from build123d import *


with BuildPart() as f1:
    # F0 (on Front) → F1 (revolve)
    with BuildSketch(Plane.XZ):
        Polygon((17.880435, -35.012588), (0, -35.012588), (0, -38.822588), (20.221465, -38.822588), align=None)
        with BuildLine():
            ThreePointArc((26.210172, 7.225862), (25.094249, 9.919939), (22.400172, 11.035862))
            Line((22.400172, 11.035862), (18.590172, 7.225862))
            Line((18.590172, 7.225862), (18.590172, -12.52082))
            Line((18.590172, -12.52082), (26.210172, -8.298599))
            Line((26.210172, -8.298599), (26.210172, 7.225862))
        make_face()
        Polygon((18.590172, -12.52082), (18.590172, 7.225862), (3.823765, -9.549403), (3.823765, -23.782769), (0, -28.126729), (0, -35.012588), (17.880435, -35.012588), (13.834589, -28.428022), (13.834589, -15.155875), align=None)
    revolve(axis=Axis((0, 0, -13.893363), (0, 0, -1)))


solid = f1.part
Verification items for the finished model (mm, model axes). A direction names the side the tool comes from. Coordinates: 2 decimals unless noted, no trailing zeros. Loops run counter-clockwise (first coordinate to the right, second up) from the corner with the lowest first, then second, coordinate; pieces in that order, holes last. Notation, with made-up numbers: (53.25, 53.5) -> (79.25, 53.5) arc R27 ccw to (79.25, 72.5) -> close; hole circle Ø8 at (16.5, -40). An arc over 180 degrees is marked (long way). Answer as a JSON object with one key per item and string values. Group by question number.
Item 1: Tool access check on faces 1 (the cylindrical face through (13.196, -4.156, -21.699)), 2 (the cylindrical face through (-0.829, 3.733, -16.766)). Record the directions out of +Z, -Z, +X, -X, +Y, -Y that give a thin tool (end or side, any length) a straight path to the whole face; none if there is none.
Item 2: Depth check by flat-ended pin: pin 1 (1.5 mm diameter, centred on y = -15, z = -3.5, fed in from -X); pin 2 (3 mm diameter, centred on y = -3, z = -22.5, fed in from -X); pin 3 (6 mm diameter, centred on y = -14, z = -30.5, fed in from +X). Enter the tip coordinate at first touch or a pass-through.
Item 3: Sectioned sample at B-B on z = -31. Record the boundary of the cut face in (x, y).
Item 4: Sectioned sample at A-A on z = -26. Record the boundary of the cut face in (x, y), plus the area to 3 significant figures.
Item 5: Mould release check, pull along X, two halves, no side actions. Record for faces 3 (the conical face through (-0.22, 1.01, -26.95)), 4 (the flat face through (0, 0, -38.823)), 5 (the cylindrical face through (14.09, -22.1, -0.43)): +X half, -X half, draft (parallel to the pull), parting line (faces both ways), or undercut.
Item 6: Scan lines: probe 1 along X at (y, z) = (0, -16); probe 2 along Y at (x, z) = (-5.5, 6.5); probe 3 along X at (y, z) = (0, -12.5). Record each from-to range of solid material in increasing order.
Evaluation:
{
 "1": {"face 1": "none", "face 2": "+Z"},
 "2": {"pin 1": "stops at x = -22", "pin 2": "stops at x = -13.75", "pin 3": "stops at x = 11.34"},
 "3": {"outline": "circle Ø30.83 at (0, 0)"},
 "4": {"outline": "circle Ø27.67 at (0, 0); hole circle Ø3.74 at (0, 0)", "area": "590 mm²"},
 "5": {"face 3": "undercut", "face 4": "draft", "face 5": "parting line"},
 "6": {"probe 1": "x = -13.83 to -3.82, 3.82 to 13.83", "probe 2": "y = -25.63 to -17.09, 17.09 to 25.63", "probe 3": "x = -18.63 to -3.82, 3.82 to 18.63"}
}
